Read the model definition and answer for the solid it produces. Units are mm, in the model's axes. A direction names the side the tool comes from. Coordinates: 2 decimals unless noted, no trailing zeros. Loops run counter-clockwise (first coordinate to the right, second up) from the corner with the lowest first, then second, coordinate; pieces in that order, holes last. Notation, with made-up numbers: (46.5, 66) - (103.5, 66) arc R19 ccw to (103.5, 100) - close; hole circle Ø4 at (27.25, -34). An arc over 180 degrees is marked (long way). Use CSV: the item, a comma, the result in double quotes.
```python
from build123d import *

# Parameters (mm, degrees)
SKETCH1_R           = 20
SKETCH1_R_2         = 18
BOSS_EXTRUDE1_DEPTH = 500
SKETCH2_R           = 18
SKETCH2_R_2         = 10
BOSS_EXTRUDE2_DEPTH = 10
SKETCH5_R           = 18
SKETCH5_R_2         = 15
BOSS_EXTRUDE3_DEPTH = 10


with BuildPart() as part:
    # Sketch1 → Boss-Extrude1 (new body)
    with BuildSketch(Plane(origin=(0, 0, 0), x_dir=(0, 0, -1), z_dir=(1, 0, 0))):
        Circle(SKETCH1_R)
        Circle(SKETCH1_R_2, mode=Mode.SUBTRACT)
    extrude(amount=BOSS_EXTRUDE1_DEPTH)

    # Sketch2 → Boss-Extrude2 (add)
    with BuildSketch(Plane.ZY):
        Circle(SKETCH2_R)
        Circle(SKETCH2_R_2, mode=Mode.SUBTRACT)
    extrude(amount=-BOSS_EXTRUDE2_DEPTH)

    # Sketch5 → Boss-Extrude3 (add)
    with BuildSketch(Plane(origin=(500, 0, 0), x_dir=(0, 0, -1), z_dir=(1, 0, 0))):
        Circle(SKETCH5_R)
        Circle(SKETCH5_R_2, mode=Mode.SUBTRACT)
    extrude(amount=-BOSS_EXTRUDE3_DEPTH)


solid = part.part
```
Q1. For a pull along X with two mould halves and no side action, classify faces 4 (the face through (490, 15, 4)), 5 (the face through (4.93, -9.76, -2.17)), 6 (the face through (500, 15, -3)) as +X half, -X half, draft (parallel to the pull), parting line (faces both ways), or undercut.
Reported:
face 4,"undercut"
face 5,"draft"
face 6,"+X half"
Q2. The part is cut by section C-C on x = 110.5. Determine the outline of the cut face in (y, z).
Reported:
outline,"circle Ø40 at (0, 0); hole circle Ø36 at (0, 0)"
Q3. Find the intervals of material crossed by probe 1 along Y at (x, z) = (495.25, 0); probe 2 along Y at (x, z) = (180, 0); probe 3 along X at (y, z) = (-12.5, 10), in increasing order. Write a range as [from, to].
Reported:
probe 1,"y = [-20, -15], [15, 20]"
probe 2,"y = [-20, -18], [18, 20]"
probe 3,"x = [0, 10], [490, 500]"
Q4. Given P1, Ø2, axis at x = 120.5, z = -4.5, coming from the +Y side; P2, Ø12, axis at x = 278.5, y = -12.5, coming from the -Z side; P3, Ø12, axis at y = 14, z = 13, coming from the -X side; P4, Ø8, axis at x = 388.5, y = 7, coming from the -Z side, each flat-ended and moving along its own axis, determine where each tip first touches the part or whether it passes through.
Reported:
P1,"stops at y = 19.69"
P2,"stops at z = -18.91"
P3,"stops at x = 0"
P4,"stops at z = -19.77"
Q5. The part is cut by section A-A on y = 0. Determine the outline of the cut face in (x, z), and give its area (3 significant figures).
Reported:
outline,"(0, -20) - (500, -20) - (500, -15) - (490, -15) - (490, -18) - (10, -18) - (10, -10) - (0, -10) - close; (0, 10) - (10, 10) - (10, 18) - (490, 18) - (490, 15) - (500, 15) - (500, 20) - (0, 20) - close"
area,"2,220 mm²"
Q6. A tool of negligible diameter and unlimited length cuts with its end or side. For faces 1 (the face through (246.64, 17.847, 2.343)), 2 (the face through (0, 9, -5)), 3 (the face through (495.07, 0.66, 14.985)), from which of +Z, -Z, +X, -X, +Y, -Y can it reach the whole face along a straight path? Write none if from no direction.
Reported:
face 1,"none"
face 2,"+Z, -Z, -X, +Y, -Y"
face 3,"+X"
